```python
from build123d import *

# Parameters (mm, degrees)
F0_R     = 8
F1_DEPTH = 14
F2_R     = 9.5
F2_R_2   = 8
F3_DEPTH = 14
F4_DEPTH = 3
F5_DEPTH = 6.2
F6_R     = 3.5
F7_DEPTH = 11.001
F9_DEPTH = 0.5


with BuildPart() as f1:
    # F0 (on Right) → F1 (new body)
    with BuildSketch(Plane.YZ):
        Circle(F0_R)
    extrude(amount=F1_DEPTH)

    # F4 (cut): a face of the model
    f4_faces = [f1.faces().sort_by_distance(p)[0] for p in [
        (14, 0, 0),
    ]]
    extrude(f4_faces, amount=-F4_DEPTH, mode=Mode.SUBTRACT)

    # F5 (cut): a face of the model
    f5_faces = [f1.faces().sort_by_distance(p)[0] for p in [
        (0, 0, 0),
    ]]
    extrude(f5_faces, amount=-F5_DEPTH, mode=Mode.SUBTRACT)

    # F6 (on face) → F7 (cut, through all)
    with BuildSketch(Plane.YZ.offset(11)):
        Circle(F6_R)
    extrude(amount=-F7_DEPTH, mode=Mode.SUBTRACT)



with BuildPart() as f3:
    # F2 (on face) → F3 (new body)
    with BuildSketch(Plane(origin=(0, 0, 0), x_dir=(0, -1, 0), z_dir=(-1, 0, 0))):
        Circle(F2_R)
        Circle(F2_R_2, mode=Mode.SUBTRACT)
    extrude(amount=-F3_DEPTH)


with BuildPart() as f1_1:
    add(f1.part)

    add(f3.part)  # F9 merges F3
    # F8 (on face) → F9 (join)
    with BuildSketch(Plane.YZ.offset(11)):
        with BuildLine():
            ThreePointArc((-3.7052864958, -3.9455150793), (-3.8272860657, -3.8272860657), (-3.9455150793, -3.7052864958))
            Line((-3.9455150793, -3.7052864958), (-5.9861921895, -5.3071181511))
            ThreePointArc((-5.9861921895, -5.3071181511), (-5.6568542495, -5.6568542495), (-5.3071181511, -5.9861921895))
            Line((-5.3071181511, -5.9861921895), (-3.7052864958, -3.9455150793))
        make_face()
        with BuildLine():
            ThreePointArc((-4.9331216086, -2.2272288729), (-5.0005902294, -2.0713122929), (-5.0631323811, -1.9133551026))
            Line((-5.0631323811, -1.9133551026), (-7.5614666316, -2.6123212626))
            ThreePointArc((-7.5614666316, -2.6123212626), (-7.3910362601, -3.0614674589), (-7.1939544103, -3.4995742515))
            Line((-7.1939544103, -3.4995742515), (-4.9331216086, -2.2272288729))
        make_face()
        with BuildLine():
            ThreePointArc((-5.4099336753, -0.1698672604), (-5.4125998612, 0), (-5.4099336753, 0.1698672604))
            Line((-5.4099336753, 0.1698672604), (-7.9855763239, 0.4801778575))
            ThreePointArc((-7.9855763239, 0.4801778575), (-8, 0), (-7.9855763239, -0.4801778575))
            Line((-7.9855763239, -0.4801778575), (-5.4099336753, -0.1698672604))
        make_face()
        with BuildLine():
            ThreePointArc((-5.0631323811, 1.9133551026), (-5.0005902294, 2.0713122929), (-4.9331216086, 2.2272288729))
            Line((-4.9331216086, 2.2272288729), (-7.1939544103, 3.4995742515))
            ThreePointArc((-7.1939544103, 3.4995742515), (-7.3910362601, 3.0614674589), (-7.5614666316, 2.6123212626))
            Line((-7.5614666316, 2.6123212626), (-5.0631323811, 1.9133551026))
        make_face()
        with BuildLine():
            ThreePointArc((-3.9455150793, 3.7052864958), (-3.8272860657, 3.8272860657), (-3.7052864958, 3.9455150793))
            Line((-3.7052864958, 3.9455150793), (-5.3071181511, 5.9861921895))
            ThreePointArc((-5.3071181511, 5.9861921895), (-5.6568542495, 5.6568542495), (-5.9861921895, 5.3071181511))
            Line((-5.9861921895, 5.3071181511), (-3.9455150793, 3.7052864958))
        make_face()
        with BuildLine():
            ThreePointArc((-2.2272288729, 4.9331216086), (-2.0713122929, 5.0005902294), (-1.9133551026, 5.0631323811))
            Line((-1.9133551026, 5.0631323811), (-2.6123212626, 7.5614666316))
            ThreePointArc((-2.6123212626, 7.5614666316), (-3.0614674589, 7.3910362601), (-3.4995742515, 7.1939544103))
            Line((-3.4995742515, 7.1939544103), (-2.2272288729, 4.9331216086))
        make_face()
        with BuildLine():
            ThreePointArc((-0.1698672604, 5.4099336753), (0, 5.4125998612), (0.1698672604, 5.4099336753))
            Line((0.1698672604, 5.4099336753), (0.4801778575, 7.9855763239))
            ThreePointArc((0.4801778575, 7.9855763239), (0, 8), (-0.4801778575, 7.9855763239))
            Line((-0.4801778575, 7.9855763239), (-0.1698672604, 5.4099336753))
        make_face()
        with BuildLine():
            Line((2.6123212626, 7.5614666316), (1.9133551026, 5.0631323811))
            ThreePointArc((1.9133551026, 5.0631323811), (2.0713122929, 5.0005902294), (2.2272288729, 4.9331216086))
            Line((2.2272288729, 4.9331216086), (3.4995742515, 7.1939544103))
            ThreePointArc((3.4995742515, 7.1939544103), (3.0614674589, 7.3910362601), (2.6123212626, 7.5614666316))
        make_face()
        with BuildLine():
            Line((5.3071181511, 5.9861921895), (3.7052864958, 3.9455150793))
            ThreePointArc((3.7052864958, 3.9455150793), (3.8272860657, 3.8272860657), (3.9455150793, 3.7052864958))
            Line((3.9455150793, 3.7052864958), (5.9861921895, 5.3071181511))
            ThreePointArc((5.9861921895, 5.3071181511), (5.6568542495, 5.6568542495), (5.3071181511, 5.9861921895))
        make_face()
        with BuildLine():
            Line((7.1939544103, 3.4995742515), (4.9331216086, 2.2272288729))
            ThreePointArc((4.9331216086, 2.2272288729), (5.0005902294, 2.0713122929), (5.0631323811, 1.9133551026))
            Line((5.0631323811, 1.9133551026), (7.5614666316, 2.6123212626))
            ThreePointArc((7.5614666316, 2.6123212626), (7.3910362601, 3.0614674589), (7.1939544103, 3.4995742515))
        make_face()
        with BuildLine():
            Line((7.9855763239, 0.4801778575), (5.4099336753, 0.1698672604))
            ThreePointArc((5.4099336753, 0.1698672604), (5.4119332737, 0.0849440915), (5.4125998612, 0))
            ThreePointArc((5.4125998612, 0), (5.4119332737, -0.0849440915), (5.4099336753, -0.1698672604))
            Line((5.4099336753, -0.1698672604), (7.9855763239, -0.4801778575))
            ThreePointArc((7.9855763239, -0.4801778575), (7.9963932679, -0.2401972196), (8, 0))
            ThreePointArc((8, 0), (7.9963932679, 0.2401972196), (7.9855763239, 0.4801778575))
        make_face()
        with BuildLine():
            Line((7.5614666316, -2.6123212626), (5.0631323811, -1.9133551026))
            ThreePointArc((5.0631323811, -1.9133551026), (5.0005902294, -2.0713122929), (4.9331216086, -2.2272288729))
            Line((4.9331216086, -2.2272288729), (7.1939544103, -3.4995742515))
            ThreePointArc((7.1939544103, -3.4995742515), (7.3910362601, -3.0614674589), (7.5614666316, -2.6123212626))
        make_face()
        with BuildLine():
            Line((5.9861921895, -5.3071181511), (3.9455150793, -3.7052864958))
            ThreePointArc((3.9455150793, -3.7052864958), (3.8272860657, -3.8272860657), (3.7052864958, -3.9455150793))
            Line((3.7052864958, -3.9455150793), (5.3071181511, -5.9861921895))
            ThreePointArc((5.3071181511, -5.9861921895), (5.6568542495, -5.6568542495), (5.9861921895, -5.3071181511))
        make_face()
        with BuildLine():
            Line((3.4995742515, -7.1939544103), (2.2272288729, -4.9331216086))
            ThreePointArc((2.2272288729, -4.9331216086), (2.0713122929, -5.0005902294), (1.9133551026, -5.0631323811))
            Line((1.9133551026, -5.0631323811), (2.6123212626, -7.5614666316))
            ThreePointArc((2.6123212626, -7.5614666316), (3.0614674589, -7.3910362601), (3.4995742515, -7.1939544103))
        make_face()
        with BuildLine():
            ThreePointArc((0.1698672604, -5.4099336753), (0, -5.4125998612), (-0.1698672604, -5.4099336753))
            Line((-0.1698672604, -5.4099336753), (-0.4801778575, -7.9855763239))
            ThreePointArc((-0.4801778575, -7.9855763239), (0, -8), (0.4801778575, -7.9855763239))
            Line((0.4801778575, -7.9855763239), (0.1698672604, -5.4099336753))
        make_face()
        with BuildLine():
            ThreePointArc((-1.9133551026, -5.0631323811), (-2.0713122929, -5.0005902294), (-2.2272288729, -4.9331216086))
            Line((-2.2272288729, -4.9331216086), (-3.4995742515, -7.1939544103))
            ThreePointArc((-3.4995742515, -7.1939544103), (-3.0614674589, -7.3910362601), (-2.6123212626, -7.5614666316))
            Line((-2.6123212626, -7.5614666316), (-1.9133551026, -5.0631323811))
        make_face()
    extrude(amount=F9_DEPTH)


solid = f1_1.part
```
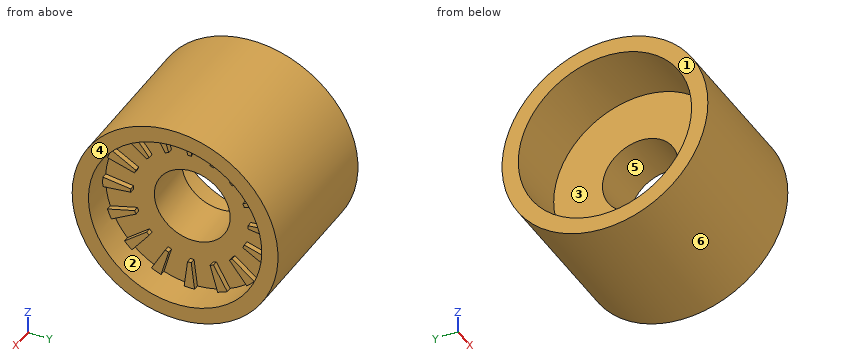
Check sheet for the modelled part. Datum: model origin and axes. Units: mm. Face numbers are marked on the shaded views. A direction names the side the tool comes from. Round coordinates to 2 decimals unless told otherwise and drop trailing zeros. Write each loop counter-clockwise with the first axis right and the second up, starting at its lowest first coordinate (ties: lowest second). Pieces come first, ordered by that corner, then holes. Notation, with made-up numbers: (5.5, -27) -> (10.5, -27) arc R22 ccw to (10.5, -7) -> close; hole circle Ø4 at (79, 47). An arc over 180 degrees is marked (long way). One line per question, with ' | ' between items. Start each with the question number.
1. Sectioned sample at B-B, the plane x = 10.5. Record the cut outline in (y, z).
2. Sectioned sample at C-C, the plane x = 3.75. Record the cut outline in (y, z), then the cut area to 3 significant figures.
3. Release check for a two-part mould opening along Z. For the marked faces 4, 5 and 6 record: +Z half, -Z half, draft (parallel to the pull), parting line (faces both ways), or undercut.
4. Depth check by flat-ended pin: pin 1 (6 mm diameter, centred on x = 2, z = 4, fed in from +Y); pin 2 (1.7 mm diameter, centred on y = -6, z = -2.5, fed in from +X); pin 3 (9.5 mm diameter, centred on y = 0, z = 0, fed in from +X). Enter the tip coordinate at first touch or a pass-through.
5. Scan lines: line 1 along Z through (x, y) = (2.5, 0); line 2 along Z through (x, y) = (9.65, 0); line 3 along X through (y, z) = (-4.75, -1.5). Record each from-to range of solid material in increasing order. Write a range as from..to.
6. Set-up check for the marked faces 1, 2 and 3: record each of +Z, -Z, +X, -X, +Y, -Y from which the full face is reachable in a straight line by a thin tool's end or side.
7. Sectioned sample at A-A, the plane z = -6.5. Record the cut outline in (x, y).
Taken from the geometry:
1) outline: circle Ø19 at (0, 0); hole circle Ø7 at (0, 0)
2) outline: circle Ø19 at (0, 0); hole circle Ø16 at (0, 0) | area: 82.5 mm^2
3) face 4: draft | face 5: undercut | face 6: parting line
4) pin 1: stops at y = 9.45 | pin 2: stops at x = 11.5 | pin 3: stops at x = 11
5) line 1: z = -9.5..-8, 8..9.5 | line 2: z = -9.5..-3.5, 3.5..9.5 | line 3: x = 6.2..11
6) face 1: +Z, -Z, -X, +Y, -Y | face 2: +X | face 3: -X
7) outline: (0, -6.93) -> (14, -6.93) -> (14, -4.66) -> (11, -4.66) -> (11, -3.11) -> (11.5, -3.11) -> (11.5, -2.32) -> (11, -2.32) -> (11, -0.3) -> (11.5, -0.3) -> (11.5, 0.3) -> (11, 0.3) -> (11, 2.32) -> (11.5, 2.32) -> (11.5, 3.11) -> (11, 3.11) -> (11, 4.66) -> (14, 4.66) -> (14, 6.93) -> (0, 6.93) -> (0, 4.66) -> (6.2, 4.66) -> (6.2, -4.66) -> (0, -4.66) -> close
